Autodesk Inventor part; units mm, degrees
ref_plane "YZ Plane" through (0, 0, 0) normal (1, 0, 0) x (0, 1, 0)
ref_plane "XZ Plane" through (0, 0, 0) normal (0, 1, 0) x (-1, 0, 0)
ref_plane "XY Plane" through (0, 0, 0) normal (0, 0, 1) x (1, 0, 0)
sketch "스케치1" plane through (0, 0, 0) normal (0, 0, 1) x (1, 0, 0)
  line L0 (0, 0) -> (47.013, 0) construction
  line L1 (0, -2.5) -> (47.013, -2.5)
  line L2 (47.013, 2.5) -> (0, 2.5)
  arc A0 (0, 2.5) -> (0, -2.5) centre (0, 0) ccw
  arc A1 (47.013, -2.5) -> (47.013, 2.5) centre (47.013, 0) ccw
  circle A2 centre (0, 0) radius 1.5
  circle A3 centre (47.013, 0) radius 1.5
  point P0 (23.5065, 0)
  point P1 (49.513, 0)
  point P2 (-2.5, 0)
  dimension "d0" = 5
  dimension "d4" = 3
  dimension "d5" = 3
  dimension "d6" = 47.013
extrude "돌출1" add sketch "스케치1" along normal blind 4
properties part number "SteeringAxis"
Input: part model. Units: mm. Frame: model coordinates. Coordinates: 2 decimals unless noted, no trailing zeros. Write each loop counter-clockwise with the first axis right and the second up, starting at its lowest first coordinate (ties: lowest second). Pieces come first, ordered by that corner, then holes. Notation, with made-up numbers: M -10.75,-4.75 L 0.25,-4.75 A23 cw 0.25,34.25 Z; hole C 10.5,-18 d4. An arc over 180 degrees is marked long. Answer as a JSON object with one key per item and string values. Group by question number.
(1) Section C-C on y = -2.05. Output: boundary loops of the cut face in (x, z), plus the area to 3 significant figures.
(2) Mould query, pull axis X, two halves, no side actions, for faces 1 (the face through (23, 0, 0)), 2 (the face through (-1.5, -0.07, 1.97)), 3 (the face through (-2.5, -0.1, 2)). Classes: pulls with the +X half, pulls with the -X half, needs draft (parallel to the pull), parting line crosses it, or undercut.
(3) Section A-A on y = 0. Output: boundary loops of the cut face in (x, z).
(4) Contact query for flat-ended pins moving along their axis: P1, Ø1, axis at y = -1, z = 3, coming from the +X side; P2, Ø2.5, axis at x = 0, y = 0, coming from the +Z side. Output: stop coordinate, or through.
(5) Ray query, line 1 along X through (y, z) = (-0.1, 2.75); line 2 along Y through (x, z) = (0, 3); line 3 along X through (y, z) = (-1.2, 2.05). Return the intervals inside material, ascending. Write a range as [from, to].
(6) Section B-B on z = 0.8. Output: boundary loops of the cut face in (x, y).
Result set:
{
 "1": {"outline": "M -1.43,0 L 48.44,0 L 48.44,4 L -1.43,4 Z", "area": "199 mm2"},
 "2": {"face 1": "needs draft", "face 2": "undercut", "face 3": "pulls with the -X half"},
 "3": {"outline": "M -2.5,0 L -1.5,0 L -1.5,4 L -2.5,4 Z; M 1.5,0 L 45.51,0 L 45.51,4 L 1.5,4 Z; M 48.51,0 L 49.51,0 L 49.51,4 L 48.51,4 Z"},
 "4": {"P1": "stops at x = 49.46", "P2": "passes through"},
 "5": {"line 1": "x = [-2.5, -1.5], [1.5, 45.52], [48.51, 49.51]", "line 2": "y = [-2.5, -1.5], [1.5, 2.5]", "line 3": "x = [-2.19, -0.9], [0.9, 46.11], [47.91, 49.21]"},
 "6": {"outline": "M 0,-2.5 L 47.01,-2.5 A2.5 ccw 47.01,2.5 L 0,2.5 A2.5 ccw Z; hole C 0,0 d3; hole C 47.01,0 d3"}
}
